Autodesk Inventor part; units mm, degrees
ref_plane "YZ Plane" through (0, 0, 0) normal (1, 0, 0) x (0, 1, 0)
ref_plane "XZ Plane" through (0, 0, 0) normal (0, 1, 0) x (-1, 0, 0)
ref_plane "XY Plane" through (0, 0, 0) normal (0, 0, 1) x (1, 0, 0)
sketch "Sketch1" plane through (0, 0, 0) normal (0, 1, 0) x (-1, 0, 0)
  line L0 (-25, 50) -> (25, 50)
  line L1 (25, 50) -> (25, -50)
  line L2 (25, -50) -> (-25, -50)
  line L3 (-25, -50) -> (-25, 50)
  line L4 (-25, 50) -> (25, -50) construction
  line L5 (25, 50) -> (-25, -50) construction
  circle A0 centre (-11, 38) radius 6.7
  circle A1 centre (-11, -38) radius 6.7
  point P0 (0, 0)
  dimension "d0" = 13.4
  dimension "d1" = 100
  dimension "d2" = 50
  dimension "d4" = 12
  dimension "d5" = 12
  dimension "d6" = 14
extrude "Extrusion1" add sketch "Sketch1" along normal blind 20
sketch "Sketch2" plane through (0, 0, 0) normal (0, -1, 0) x (1, 0, 0)
  circle A0 centre (-15, -30) radius 2.65
  circle A1 centre (-15, 30) radius 2.65
  line L0 (-25, -50) -> (-25, 50)
  line L1 (25, -50) -> (-25, -50)
  line L2 (-25, 50) -> (25, 50)
  point P0 (0, 0)
  dimension "d9" = 5.3
  dimension "d10" = 10
  dimension "d11" = 20
  dimension "d12" = 20
  dimension "d13" = 10
extrude "Extrusion2" cut sketch "Sketch2" against normal through all
sketch "Sketch3" plane through (0, 0, 0) normal (0, -1, 0) x (1, 0, 0)
  line L0 (25, 50) -> (25, -50)
  line L1 (-25, 50) -> (25, 50)
  line L2 (25, -50) -> (24, -50)
  line L3 (24, -50) -> (24, 50)
  line L4 (24, 50) -> (25, 50)
  line L5 (25, 50) -> (25, -50)
  point P0 (0, 0)
  dimension "d16" = 1
extrude "Extrusion3" cut sketch "Sketch3" against normal through all
fillet "Fillet1" radius 5 2 edges at (-25, 10, 50) (-25, 10, -50)
sketch "Sketch4" plane through (0, 0, 0) normal (0, -1, 0) x (1, 0, 0)
  circle A0 centre (-15, -30) radius 2.65
  circle A1 centre (-15, -30) radius 4.1
  circle A2 centre (-15, 30) radius 2.65
  circle A3 centre (-15, 30) radius 4.1
  line L0 (-19.7343, -30) -> (-17.3671, -25.9)
  line L1 (-17.3671, -25.9) -> (-12.6329, -25.9)
  line L2 (-12.6329, -25.9) -> (-10.2657, -30)
  line L3 (-10.2657, -30) -> (-12.6329, -34.1)
  line L4 (-12.6329, -34.1) -> (-17.3671, -34.1)
  line L5 (-17.3671, -34.1) -> (-19.7343, -30)
  line L6 (-19.7311, 29.8275) -> (-17.5149, 34.011)
  line L7 (-17.5149, 34.011) -> (-12.7838, 34.1835)
  line L8 (-12.7838, 34.1835) -> (-10.2689, 30.1725)
  line L9 (-10.2689, 30.1725) -> (-12.4851, 25.989)
  line L10 (-12.4851, 25.989) -> (-17.2162, 25.8165)
  line L11 (-17.2162, 25.8165) -> (-19.7311, 29.8275)
  point P0 (0, 0)
  dimension "d20" = 8.2
  dimension "d21" = 8.2
extrude "Extrusion4" [suppressed]
sketch "Sketch5" plane through (0, 0, 0) normal (0, -1, 0) x (1, 0, 0)
  circle A0 centre (11, 0) radius 4.15
  circle A1 centre (11, -38) radius 6.7
  point P0 (0, 0)
  dimension "d24" = 8.3
extrude "Extrusion5" cut sketch "Sketch5" against normal through all contours A0
sketch "Sketch6" plane through (24, 0, 50) normal (1, 0, 0) x (0, 0, -1)
  line L0 (57.05, 6.9) -> (42.95, 6.9)
  line L1 (42.95, 6.9) -> (42.95, 13.1)
  line L2 (42.95, 13.1) -> (57.05, 13.1)
  line L3 (57.05, 13.1) -> (57.05, 6.9)
  line L4 (57.05, 6.9) -> (42.95, 13.1) construction
  line L5 (42.95, 6.9) -> (57.05, 13.1) construction
  line L6 (0, 20) -> (100, 20)
  point P0 (50, 0)
  point P1 (50, 10)
  dimension "d27" = 10
  dimension "d28" = 14.1
  dimension "d29" = 6.2
extrude "Extrusion6" cut sketch "Sketch6" against normal blind 22
fillet "Fillet2" radius 5 2 edges at (24, 10, -50) (24, 10, 50)
sketch "Sketch7" plane through (0, 0, 0) normal (0, -1, 0) x (1, 0, 0)
  circle A0 centre (-15, -30) radius 2.65
  circle A1 centre (-15, -30) radius 4.5
  circle A2 centre (-15, 30) radius 2.65
  circle A3 centre (-15, 30) radius 4.5
  point P0 (0, 0)
  dimension "d35" = 9
extrude "Extrusion7" cut sketch "Sketch7" against normal blind 5 contours A1 | A2 | A3
properties part number "Movingjaw"
CAD build for the part. Positions are in the model's coordinates, mm. A direction names the side the tool comes from. Coordinates: 2 decimals unless noted, no trailing zeros. Write each loop counter-clockwise with the first axis right and the second up, starting at its lowest first coordinate (ties: lowest second). Pieces come first, ordered by that corner, then holes. Notation, with made-up numbers: (16, -37) -> (60, -37) arc R14 ccw to (60, -22) -> close; hole circle Ø10 at (78.25, 61). An arc over 180 degrees is marked (long way). Return JSON: item names as keys, results as strings. Group by question number.
Q1. Cut at B-B, the plane z = 38. Give the cut face in (x, y), then the cut area to 3 significant figures.
Q2. Drill centre lines: line 1 (Z direction, x = 11, y = 4.5); line 2 (Z direction, x = 11, y = 12); line 3 (Z direction, x = -15, y = 9). Where is each one in solid material? Low to high.
Q3. Cut at C-C, the plane y = 8.5. Give the cut face in (x, z).
Q4. Flat gauge pins, fed straight in: pin 1 (4.5 mm diameter, centred on x = -16.5, z = -31.5, fed in from -Y); pin 2 (3 mm diameter, centred on x = -15, z = 30, fed in from +Y); pin 3 (3 mm diameter, centred on y = 11, z = 3, fed in from +X); pin 4 (15.5 mm diameter, centred on x = 9, z = 0, fed in from -Y). Where does each tip first touch, or does it go through?
Q5. Which spindle directions (+Z, -Z, +X, -X, +Y, -Y) get a long thin tool onto all of the face, cutting with end or side? Do faces 5 (the face through (-23, 10, -49)), 6 (the face through (-13, 5, 28)), 7 (the face through (16, 6.9, 0)). Say none if no direction does.
Q6. Cut at A-A, the plane x = 11. Give the cut face in (y, z).
Q7. Cut at D-D, the plane y = 1.75. Give the cut face in (x, z), then the cut area to 3 significant figures.
Q8. Pull direction Y, two halves, no side cores. Call faces 1 (the face through (16, 13.1, 0)), 2 (the face through (-13, 5, -32)), 3 (the face through (-25, 10, 1)), 4 (the face through (0, 20, 1)): released by +Y, released by -Y, zero draft, split by the parting line, or undercut.
Returned:
{
 "1": {"outline": "(-25, 0) -> (4.3, 0) -> (4.3, 20) -> (-25, 20) -> close; (17.7, 0) -> (24, 0) -> (24, 20) -> (17.7, 20) -> close", "area": "712 mm2"},
 "2": {"line 1": "z = -50 to -44.7, -31.3 to -4.15, 4.15 to 31.3, 44.7 to 50", "line 2": "z = -50 to -44.7, -31.3 to -7.05, 7.05 to 31.3, 44.7 to 50", "line 3": "z = -50 to -32.65, -27.35 to 27.35, 32.65 to 50"},
 "3": {"outline": "(-25, -45) arc R5 ccw to (-20, -50) -> (19, -50) arc R5 ccw to (24, -45) -> (24, -7.05) -> (2, -7.05) -> (2, 7.05) -> (24, 7.05) -> (24, 45) arc R5 ccw to (19, 50) -> (-20, 50) arc R5 ccw to (-25, 45) -> close; hole circle Ø5.3 at (-15, -30); hole circle Ø5.3 at (-15, 30); hole circle Ø13.4 at (11, -38); hole circle Ø13.4 at (11, 38)"},
 "4": {"pin 1": "stops at y = 5", "pin 2": "passes through", "pin 3": "stops at x = 2", "pin 4": "stops at y = 0"},
 "5": {"face 5": "-Z, -X, +Y, -Y", "face 6": "-Y", "face 7": "+X"},
 "6": {"outline": "(0, -50) -> (20, -50) -> (20, -44.7) -> (0, -44.7) -> close; (0, -31.3) -> (20, -31.3) -> (20, -4.15) -> (13.1, -4.15) -> (13.1, -7.05) -> (6.9, -7.05) -> (6.9, -4.15) -> (0, -4.15) -> close; (0, 4.15) -> (6.9, 4.15) -> (6.9, 7.05) -> (13.1, 7.05) -> (13.1, 4.15) -> (20, 4.15) -> (20, 31.3) -> (0, 31.3) -> close; (0, 44.7) -> (20, 44.7) -> (20, 50) -> (0, 50) -> close"},
 "7": {"outline": "(-25, -45) arc R5 ccw to (-20, -50) -> (19, -50) arc R5 ccw to (24, -45) -> (24, 45) arc R5 ccw to (19, 50) -> (-20, 50) arc R5 ccw to (-25, 45) -> close; hole circle Ø9 at (-15, -30); hole circle Ø9 at (-15, 30); hole circle Ø13.4 at (11, -38); hole circle Ø13.4 at (11, 38); hole circle Ø8.3 at (11, 0)", "area": "4,420 mm2"},
 "8": {"face 1": "undercut", "face 2": "released by -Y", "face 3": "zero draft", "face 4": "released by +Y"}
}
